The listing builds one solid part. Answer for the finished solid, in the listing's coordinates (mm). Round coordinates to 2 decimals unless told otherwise and drop trailing zeros. Write each loop counter-clockwise with the first axis right and the second up, starting at its lowest first coordinate (ties: lowest second). Pieces come first, ordered by that corner, then holes. Notation, with made-up numbers: (25.5, 60.25) - (74.5, 60.25) arc R30 cw to (74.5, 90.25) - close; hole circle Ø2 at (74, -9.5). An arc over 180 degrees is marked (long way). Use a Markdown table: item, result. Add a question column.
1) A cutting plane is placed at A-A (y = -6). Give the vertices of the cut face in (x, z), then the cut area to 3 significant figures.
2) A cutting plane is placed at C-C (z = 2.15). State how many separate pieces and enclosed holes the cut face has, then the cut area to 3 significant figures.
3) A cutting plane is placed at B-B (x = 14). Give the vertices of the cut face in (y, z).
4) Find the intervals of material crossed by probe 1 along Y at (x, z) = (31, 0.9) (3 decimals); probe 2 along X at (y, z) = (-5, 1.15); probe 3 along Y at (x, z) = (67.5, 1.15) (3 decimals), in increasing order. Write a range as from..to.
5) Each of these flat-tipped pins is pushed along its axis until it touches: P1, Ø3.5, axis at x = 67.5, y = -15, coming from the +Z side; P2, Ø1.5, axis at x = 35.5, z = 2, coming from the -Y side; P3, Ø1.8, axis at x = -31, y = -25, coming from the -Z side. Where does it stop, or does it pass through?
6) A cutting plane is placed at D-D (y = 25). Give the vertices of the cut face in (x, z) (3 decimals), then the cut area to 3 significant figures.
```python
from build123d import *

# Parameters (mm, degrees)
SKETCH_1_R          = 1.525
EXTRUDE_1_DEPTH     = 3
CUT_EXTRUDE_1_DEPTH = 3
CUT_EXTRUDE_2_DEPTH = 3
FILLET_1_R          = 1.6


with BuildPart() as part:
    # 草图1 → 凸台-拉伸1 (new body)
    with BuildSketch(Plane.XY):
        Polygon((-70.5, 17.288636625), (-31.403523682, 28), (31.403523682, 28), (70.5, 17.288636625), (70.5, -17.288636625), (31.403523682, -28), (-31.403523682, -28), (-70.5, -17.288636625), align=None)
        with Locations((31, 25)):
            Circle(SKETCH_1_R, mode=Mode.SUBTRACT)
        with Locations((-31, 25)):
            Circle(SKETCH_1_R, mode=Mode.SUBTRACT)
        with Locations((-31, -25)):
            Circle(SKETCH_1_R, mode=Mode.SUBTRACT)
        with Locations((31, -25)):
            Circle(SKETCH_1_R, mode=Mode.SUBTRACT)
        with Locations((-67.5, -15)):
            Circle(SKETCH_1_R, mode=Mode.SUBTRACT)
        with Locations((-67.5, 15)):
            Circle(SKETCH_1_R, mode=Mode.SUBTRACT)
        with Locations((67.5, 15)):
            Circle(SKETCH_1_R, mode=Mode.SUBTRACT)
        with Locations((67.5, -15)):
            Circle(SKETCH_1_R, mode=Mode.SUBTRACT)
    extrude(amount=EXTRUDE_1_DEPTH)

    # 草图2 → 切除-拉伸1 (cut)
    with BuildSketch(Plane.XY.offset(3)):
        Polygon((-28, 21.058820972), (-28, -21.058820972), (-2.363174469, 0), align=None)
        Polygon((0, -1.941179028), (-25.636825531, -23), (25.636825531, -23), align=None)
        Polygon((28, 21.058820972), (2.363174469, 0), (28, -21.058820972), align=None)
        Polygon((-25.636825531, 23), (0, 1.941179028), (25.636825531, 23), align=None)
    extrude(amount=-CUT_EXTRUDE_1_DEPTH, mode=Mode.SUBTRACT)

    # 草图3 → 切除-拉伸2 (cut)
    with BuildSketch(Plane.XY.offset(3)):
        Polygon((34, 21.067527758), (34, -21.067527758), (64.5, -12.711363375), (64.5, 12.711363375), align=None)
        Polygon((-64.5, 12.711363375), (-34, 21.067527758), (-34, -21.067527758), (-64.5, -12.711363375), align=None)
    extrude(amount=-CUT_EXTRUDE_2_DEPTH, mode=Mode.SUBTRACT)

    # 圆角1
    fillet_1_edges = [part.edges().sort_by_distance(p)[0] for p in [
        (34, 21.067527758, 1.5),
        (64.5, 12.711363375, 1.5),
        (64.5, -12.711363375, 1.5),
        (34, -21.067527758, 1.5),
        (-34, 21.067527758, 1.5),
        (-34, -21.067527758, 1.5),
        (-64.5, -12.711363375, 1.5),
        (-64.5, 12.711363375, 1.5),
        (-70.5, 17.288636625, 1.5),
        (-31.403523682, 28, 1.5),
        (31.403523682, 28, 1.5),
        (70.5, 17.288636625, 1.5),
        (70.5, -17.288636625, 1.5),
        (31.403523682, -28, 1.5),
        (-31.403523682, -28, 1.5),
        (-70.5, -17.288636625, 1.5),
        (2.363174469, 0, 1.5),
        (28, 21.058820972, 1.5),
        (28, -21.058820972, 1.5),
        (-25.636825531, -23, 1.5),
        (0, -1.941179028, 1.5),
        (25.636825531, -23, 1.5),
        (0, 1.941179028, 1.5),
        (-25.636825531, 23, 1.5),
        (25.636825531, 23, 1.5),
        (-28, -21.058820972, 1.5),
        (-28, 21.058820972, 1.5),
        (-2.363174469, 0, 1.5),
    ]]
    fillet(fillet_1_edges, radius=FILLET_1_R)


solid = part.part
```
Entries:
| question | item | result |
|---|---|---|
| 1 | outline | (-70.5, 0) - (-64.5, 0) - (-64.5, 3) - (-70.5, 3) - close; (-34, 0) - (-28, 0) - (-28, 3) - (-34, 3) - close; (-9.67, 0) - (-4.94, 0) - (-4.94, 3) - (-9.67, 3) - close; (4.94, 0) - (9.67, 0) - (9.67, 3) - (4.94, 3) - close; (28, 0) - (34, 0) - (34, 3) - (28, 3) - close; (64.5, 0) - (70.5, 0) - (70.5, 3) - (64.5, 3) - close |
| 1 | area | 100 mm² |
| 2 | separate pieces | 1 |
| 2 | enclosed holes | 14 |
| 2 | area | 2,810 mm² |
| 3 | outline | (-28, 0) - (-23, 0) - (-23, 3) - (-28, 3) - close; (-13.44, 0) - (-9.56, 0) - (-9.56, 3) - (-13.44, 3) - close; (9.56, 0) - (13.44, 0) - (13.44, 3) - (9.56, 3) - close; (23, 0) - (28, 0) - (28, 3) - (23, 3) - close |
| 4 | probe 1 | y = -28..-26.525, -23.475..23.475, 26.525..28 |
| 4 | probe 2 | x = -70.5..-64.5, -34..-28, -8.45..-3.72, 3.72..8.45, 28..34, 64.5..70.5 |
| 4 | probe 3 | y = -18.111..-16.525, -13.475..13.475, 16.525..18.111 |
| 5 | P1 | stops at z = 3 |
| 5 | P2 | stops at y = -27.08 |
| 5 | P3 | passes through |
| 6 | outline | (-42.354, 0) - (-32.525, 0) - (-32.525, 3) - (-42.354, 3) - close; (-29.475, 0) - (29.475, 0) - (29.475, 3) - (-29.475, 3) - close; (32.525, 0) - (42.354, 0) - (42.354, 3) - (32.525, 3) - close |
| 6 | area | 236 mm² |
